Autodesk Inventor part; units mm, degrees
ref_plane "YZ Plane" through (0, 0, 0) normal (1, 0, 0) x (0, 1, 0)
ref_plane "XZ Plane" through (0, 0, 0) normal (0, 1, 0) x (-1, 0, 0)
ref_plane "XY Plane" through (0, 0, 0) normal (0, 0, 1) x (1, 0, 0)
sketch "Skizze1" plane through (0, 0, 0) normal (0, 0, 1) x (1, 0, 0)
  circle A0 centre (0, 0) radius 6
  dimension "d0" = 12
extrude "Extrusion1" add sketch "Skizze1" along normal blind 310
sketch "Skizze2" plane through (0, 0, 0) normal (0, 0, -1) x (-1, 0, 0)
  circle A0 centre (0, 0) radius 6
  circle A1 centre (0, 0) radius 5
  dimension "d3" = 10
extrude "Extrusion2" cut sketch "Skizze2" against normal through all
sketch "Skizze3" plane through (0, 0, 310) normal (0, 0, 1) x (1, 0, 0)
  circle A0 centre (0, 0) radius 5
  circle A1 centre (0, 0) radius 4.5
  dimension "d6" = 9
extrude "Extrusion3" cut sketch "Skizze3" against normal blind 50
hole "Bohrung1" at (0, 0, 0) direction (0, 0, 1) diameter 4.134 depth 12 tip angle 118
hole "Bohrung2" at (0, 0, 310) direction (0, 0, -1) diameter 3.242 depth 13 tip angle 118
properties part number "13_0204_022"
Build history of the part. All positions in model axes, mm. A direction names the side the tool comes from. Coordinates: 2 decimals unless noted, no trailing zeros. Order: outer loops, then holes, each group sorted by start corner. A loop starts at its lowest first (then second) coordinate and runs counter-clockwise, first axis right, second up. Notation, with made-up numbers: (-39, -21) - (-12, -21) arc R31 cw to (-12, 4) - close; hole circle Ø8 at (33.25, 41). An arc over 180 degrees is marked (long way). Write item = value, one per line. Start each with the question number.
1) 3-axis set-ups, long thin cutter, end or side, ignore diameter. For faces 1 (the face through (-0.59, 4.46, 285.35)), 2 (the face through (0, -2, 310)): which of +Z, -Z, +X, -X, +Y, -Y reach the whole face in a straight line?
2) Wall check: line 1 along Y through (x, z) = (0, 301.25); line 2 along Y through (x, z) = (0, 9.75); line 3 along Z through (x, y) = (-4.25, -2.25). Give the ranges that are in metal, low to high. Write a range as from..to.
3) Saw through at A-A on z = 59. Write the cut outline in (x, y).
4) Flat gauge pins, fed straight in: pin 1 Ø2 at (x, z) = (1.5, 195) entering from -Y; pin 2 Ø5 at (x, z) = (3.5, 230.5) entering from -Y; pin 3 Ø4 at (x, y) = (0, 0) entering from -Z. Where does each tip first touch, or does it go through?
From the geometry:
q1.face_1 = +Z
q1.face_2 = +Z, +X, -X, +Y, -Y
q2.line_1 = -4.5..-1.62, 1.62..4.5
q2.line_2 = -5..-2.07, 2.07..5
q2.line_3 = 0..260
q3.outline = circle Ø10 at (0, 0)
q4.pin_1 = -4.97
q4.pin_2 = -4.9
q4.pin_3 = 12.04
